```python
from build123d import *

# Parameters (mm, degrees)
ESBO_O1_R                = 3
ESBO_O1_R_2              = 1.6
ESBO_O1_W                = 15
ESBO_O1_H                = 3
ESBO_O1_W_2              = 42
ESBO_O1_H_2              = 21
ESBO_O1_R_3              = 9.5
ESBO_O1_H_3              = 6
RESSALTO_EXTRUS_O1_DEPTH = 6
FILETE1_R                = 5


with BuildPart() as part:
    # Esboço1 → Ressalto-extrusão1 (new body)
    with BuildSketch(Plane.XZ.offset(6)):
        with BuildLine():
            ThreePointArc((28.221137594, -123.946334359), (26.32780231, -130.898758331), (30.793557575, -136.55366306))
            Line((30.793557575, -136.55366306), (52.89462836, -146.829127406))
            ThreePointArc((52.89462836, -146.829127406), (53.923154275, -147.177291613), (55.00259, -147.2952))
            Line((55.00259, -147.2952), (102.35259, -147.2952))
            ThreePointArc((102.35259, -147.2952), (105.888123906, -145.830733906), (107.35259, -142.2952))
            Line((107.35259, -142.2952), (107.35259, -122.2))
            ThreePointArc((107.35259, -122.2), (105.888123906, -118.664466094), (102.35259, -117.2))
            Line((102.35259, -117.2), (88.05, -117.2))
            ThreePointArc((88.05, -117.2), (84.514466094, -115.735533906), (83.05, -112.2))
            Line((83.05, -112.2), (83.05, -111.6301581))
            Line((83.05, -111.6301581), (93.187089706, -99.009861475))
            ThreePointArc((93.187089706, -99.009861475), (94.95, -94), (93.187089706, -88.990138525))
            Line((93.187089706, -88.990138525), (87.547626436, -81.969218188))
            Line((87.547626436, -81.969218188), (103.678862406, -64.053665641))
            ThreePointArc((103.678862406, -64.053665641), (103.086748653, -52.755462186), (91.788545198, -53.347575939))
            Line((91.788545198, -53.347575939), (85.037246259, -60.845653032))
            ThreePointArc((85.037246259, -60.845653032), (83.355205347, -62.067727288), (81.321522132, -62.5))
            Line((81.321522132, -62.5), (53.85, -62.5))
            ThreePointArc((53.85, -62.5), (50.314466094, -63.964466094), (48.85, -67.5))
            Line((48.85, -67.5), (48.85, -76.3698419))
            Line((48.85, -76.3698419), (38.712910294, -88.990138525))
            ThreePointArc((38.712910294, -88.990138525), (36.95, -94), (38.712910294, -99.009861475))
            Line((38.712910294, -99.009861475), (44.352373564, -106.030781812))
            Line((44.352373564, -106.030781812), (28.221137594, -123.946334359))
        make_face()
        with Locations(Location((34.166296198, -129.29937921, 0), (0, 0, 270))):
            Circle(ESBO_O1_R, mode=Mode.SUBTRACT)
        with Locations(Location((51.25259, -136.7952, 0), (0, 0, 270))):
            Circle(ESBO_O1_R_2, mode=Mode.SUBTRACT)
        with Locations(Location((51.25259, -126.7952, 0), (0, 0, 270))):
            Circle(ESBO_O1_R_2, mode=Mode.SUBTRACT)
        with Locations((65.95, -115.7)):
            Rectangle(ESBO_O1_W, ESBO_O1_H, mode=Mode.SUBTRACT)
        with Locations((65.95, -106.5)):
            Rectangle(ESBO_O1_W, ESBO_O1_H, mode=Mode.SUBTRACT)
        with Locations((76.00259, -131.7952)):
            Rectangle(ESBO_O1_W_2, ESBO_O1_H_2, mode=Mode.SUBTRACT)
        with Locations(Location((100.75259, -136.7952, 0), (0, 0, 270))):
            Circle(ESBO_O1_R_2, mode=Mode.SUBTRACT)
        with Locations(Location((100.75259, -126.7952, 0), (0, 0, 270))):
            Circle(ESBO_O1_R_2, mode=Mode.SUBTRACT)
        with Locations(Location((65.95, -94, 0), (0, 0, 270))):
            Circle(ESBO_O1_R_3, mode=Mode.SUBTRACT)
        with Locations((65.95, -70.5)):
            Rectangle(ESBO_O1_W, ESBO_O1_H_3, mode=Mode.SUBTRACT)
        with Locations(Location((97.733703802, -58.70062079, 0), (0, 0, 270))):
            Circle(ESBO_O1_R, mode=Mode.SUBTRACT)
        with Locations(Location((44.95, -94, 0), (0, 0, 270))):
            Circle(ESBO_O1_R_2, mode=Mode.SUBTRACT)
        with Locations(Location((86.95, -94, 0), (0, 0, 270))):
            Circle(ESBO_O1_R_2, mode=Mode.SUBTRACT)
    extrude(amount=-RESSALTO_EXTRUS_O1_DEPTH)

    # Filete1
    # the kernel refuses this fillet: 5 mm, written as the material it adds along each edge
    with BuildSketch(Plane(origin=(83.05, -6, -111.6301581), x_dir=(0, 0, -1), z_dir=(0, 1, 0))) as filete1_piece_1:
        with BuildLine():
            CenterArc((2.031271709, -4.78165483), FILETE1_R, 106.994862895, 21.777857611)
            Line((-1.099891712, -0.883473763), (-1.162514981, -0.805510142))
            Line((-1.162514981, -0.805510142), (-0.062623268, 0.077963621))
            Line((-0.062623268, 0.077963621), (0, 0.1))
            ThreePointArc((0, 0.1), (0.28492095, 0.1), (0.540613304, 0.095633097))
            Line((0.540613304, 0.095633097), (0.5698419, 0))
        make_face()
    extrude(amount=6)
    with BuildSketch(Plane(origin=(87.547626436, -6, -81.969218188), x_dir=(0.626232684317403, 0, -0.7796362133024736), z_dir=(0, 1, 0)), Plane(origin=(44.352373564, -6, -106.030781812), x_dir=(-0.6262326843177314, 0, 0.7796362133022096), z_dir=(0, 1, 0))) as filete1_piece_2:
        with BuildLine():
            CenterArc((FILETE1_R * 0.85065630428, -FILETE1_R), FILETE1_R, 90, 80.772720506)
            Line((-FILETE1_R * 0.136403726762, -FILETE1_R * 0.839648838109), (-FILETE1_R * 0.156144927382, -FILETE1_R * 0.836441814871))
            Line((-FILETE1_R * 0.156144927382, -FILETE1_R * 0.836441814871), (-FILETE1_R * 0.0170131260856, FILETE1_R * 0.02))
            Line((-FILETE1_R * 0.0170131260856, FILETE1_R * 0.02), (FILETE1_R * 0.85065630428, FILETE1_R * 0.02))
            Line((FILETE1_R * 0.85065630428, FILETE1_R * 0.02), (FILETE1_R * 0.85065630428, 0))
        make_face()
    extrude(amount=6)
    with BuildSketch(Plane(origin=(48.85, -6, -76.3698419), x_dir=(0, 0, 1), z_dir=(0, 1, 0))) as filete1_piece_3:
        with BuildLine():
            CenterArc((FILETE1_R * 0.351888031743, -FILETE1_R), FILETE1_R, 90, 38.772720506)
            Line((-FILETE1_R * 0.274344652575, -FILETE1_R * 0.220363786698), (-FILETE1_R * 0.286869306261, -FILETE1_R * 0.204771062432))
            Line((-FILETE1_R * 0.286869306261, -FILETE1_R * 0.204771062432), (-FILETE1_R * 0.00703776063486, FILETE1_R * 0.02))
            Line((-FILETE1_R * 0.00703776063486, FILETE1_R * 0.02), (FILETE1_R * 0.351888031743, FILETE1_R * 0.02))
            Line((FILETE1_R * 0.351888031743, FILETE1_R * 0.02), (FILETE1_R * 0.351888031743, 0))
        make_face()
    extrude(amount=6)


solid = part.part
```
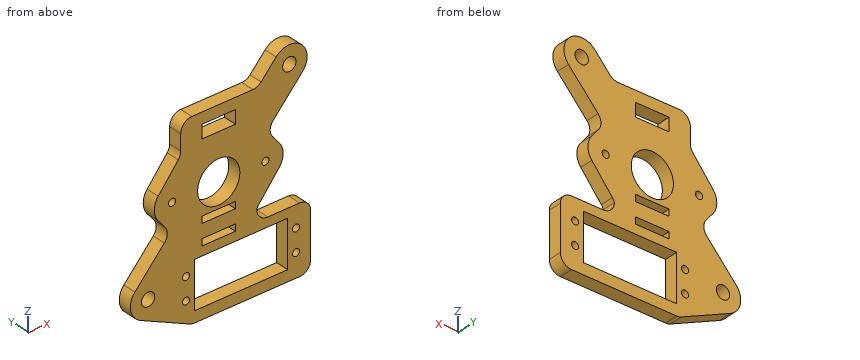
Build history of the part. All positions in model axes, mm. Round coordinates to 2 decimals unless told otherwise and drop trailing zeros. Order: outer loops, then holes, each group sorted by start corner. A loop starts at its lowest first (then second) coordinate and runs counter-clockwise, first axis right, second up. Notation, with made-up numbers: (63.5, -31.75) - (89.5, -31.75) arc R15 ccw to (89.5, -6.75) - close; hole circle Ø9 at (42, 64). An arc over 180 degrees is marked (long way). Use a Markdown table: item, result.
1) Saw through at C-C on x = 44.95. Write the cut outline in (y, z), and give its area (3 significant figures).
Recorded:
| item | result |
|---|---|
| outline | (-6, -143.14) - (0, -143.14) - (0, -95.6) - (-6, -95.6) - close; (-6, -92.4) - (0, -92.4) - (0, -81.23) - (-6, -81.23) - close |
| area | 352 mm² |
2) Wall check: L1, parallel to X at y = -3.1, z = -94; L2, parallel to X at y = -4.7, z = -129.5; L3, parallel to Z at x = 81, y = -1.7. Give the ranges that are in metal, low to high.
Recorded:
| item | result |
|---|---|
| L1 | x = 36.95 to 43.35, 46.55 to 56.45, 75.45 to 85.35, 88.55 to 94.95 |
| L2 | x = 26.17 to 31.17, 37.16 to 55, 97 to 107.35 |
| L3 | z = -147.3 to -142.3, -121.3 to -62.5 |
3) Saw through at B-B on x = 64. Write the cut outline in (y, z).
Recorded:
| item | result |
|---|---|
| outline | (-6, -147.3) - (0, -147.3) - (0, -142.3) - (-6, -142.3) - close; (-6, -121.3) - (0, -121.3) - (0, -117.2) - (-6, -117.2) - close; (-6, -114.2) - (0, -114.2) - (0, -108) - (-6, -108) - close; (-6, -105) - (0, -105) - (0, -103.3) - (-6, -103.3) - close; (-6, -84.7) - (0, -84.7) - (0, -73.5) - (-6, -73.5) - close; (-6, -67.5) - (0, -67.5) - (0, -62.5) - (-6, -62.5) - close |
4) Saw through at D-D on y = -4.4. Give the number of separate pieces and of enclosed holes in the cut face, and give its area (3 significant figures).
Recorded:
| item | result |
|---|---|
| separate pieces | 1 |
| enclosed holes | 13 |
| area | 3,650 mm² |
5) Saw through at A-A on z = -94. Write the cut outline in (x, y), and give its area (3 significant figures).
Recorded:
| item | result |
|---|---|
| outline | (36.95, -6) - (43.35, -6) - (43.35, 0) - (36.95, 0) - close; (46.55, -6) - (56.45, -6) - (56.45, 0) - (46.55, 0) - close; (75.45, -6) - (85.35, -6) - (85.35, 0) - (75.45, 0) - close; (88.55, -6) - (94.95, -6) - (94.95, 0) - (88.55, 0) - close |
| area | 196 mm² |
6) Flat gauge pins, fed straight in: pin 1 Ø5 at (x, z) = (34.17, -129.3) entering from -Y; pin 2 Ø3 at (y, z) = (-4, -104.5) entering from +X; pin 3 Ø2 at (y, z) = (-5, -117) entering from -X; pin 4 Ø3 at (x, y) = (78, -3) entering from +Z. Where does each tip first touch, or does it go through?
Recorded:
| item | result |
|---|---|
| pin 1 | passes through |
| pin 2 | stops at x = 89.98 |
| pin 3 | stops at x = 33.58 |
| pin 4 | stops at z = -62.5 |
